Model file for the job. Use its own axes, mm. Coordinates: 2 decimals unless noted, no trailing zeros. Loops run counter-clockwise (first coordinate to the right, second up) from the corner with the lowest first, then second, coordinate; pieces in that order, holes last.
from build123d import *

# Parameters (mm, degrees)
SKETCH1_W           = 308.670974492
SKETCH1_H           = 266.7
SKETCH1_R           = 14.2875
SKETCH1_R_2         = 14.2621
SKETCH1_R_3         = 15.365901376
BOSS_EXTRUDE1_DEPTH = 5.08


with BuildPart() as part:
    # Sketch1 → Boss-Extrude1 (new body)
    with BuildSketch(Plane.XY):
        with Locations((-73.533038571, -40.364359579)):
            Rectangle(SKETCH1_W, SKETCH1_H)
        Circle(SKETCH1_R, mode=Mode.SUBTRACT)
        with Locations((-138.201859455, -157.325049094)):
            Circle(SKETCH1_R, mode=Mode.SUBTRACT)
        with Locations((-166.847551324, 48.535640421)):
            Circle(SKETCH1_R_2, mode=Mode.SUBTRACT)
        with Locations((-166.847551324, -141.964359579)):
            Circle(SKETCH1_R_3, mode=Mode.SUBTRACT)
        with Locations((-116.047551324, -135.614359579)):
            Circle(SKETCH1_R_2, mode=Mode.SUBTRACT)
        with Locations((-65.247551325, -103.864359579)):
            Circle(SKETCH1_R_2, mode=Mode.SUBTRACT)
        with Locations((-14.447551325, -97.514359579)):
            Circle(SKETCH1_R_2, mode=Mode.SUBTRACT)
        with Locations((36.352448675, -94.389320601)):
            Circle(SKETCH1_R, mode=Mode.SUBTRACT)
    extrude(amount=BOSS_EXTRUDE1_DEPTH)


solid = part.part
Q1. Slice it at A-A (y = 0). List the corners of the cut face in (x, z).
Answers:
outline: (-227.87, 0) - (-14.29, 0) - (-14.29, 5.08) - (-227.87, 5.08) - close; (14.29, 0) - (80.8, 0) - (80.8, 5.08) - (14.29, 5.08) - close
Q2. Mould opens along Y. For faces 1 (the flat face through (-76, -38, 5.08)), 2 (the cylindrical face through (33.26, -108.34, 2.5)) say: +Y half, -Y half, draft (parallel to the pull), parting line (faces both ways), or undercut.
Answers:
face 1: draft
face 2: undercut
Q3. Slice it at B-B (z = 1.5). Count the separate pieces of the cut face and the enclosed holes in it, and give its area (3 significant figures).
Answers:
separate pieces: 1
enclosed holes: 8
area: 77,100 mm2
Q4. Drill centre lines: line 1 (Y direction, x = -167, z = 0.75); line 2 (X direction, y = -128, z = 2.7); line 3 (Y direction, x = -8, z = 3.8). Where is each one in solid material? Low to high.
Answers:
line 1: y = -173.71 to -157.33, -126.6 to 34.27, 62.8 to 92.99
line 2: x = -227.87 to -173.26, -160.44 to -128.11, -103.99 to 80.8
line 3: y = -173.71 to -110.24, -84.79 to -11.84, 11.84 to 92.99
Q5. Flat gauge pin, fed straight in: P1, Ø23, axis at x = -166.85, y = 48.54, coming from the -Z side. Where does the tip first touch, or does it go through?
Answers:
P1: passes through
